Here's how the part is built. I have some questions about the finished solid (model axes, mm). A direction names the side the tool comes from. Give positions to 0.01 mm unless a question says otherwise; leave off trailing zeros. Write each loop counter-clockwise with the first axis right and the second up, starting at its lowest first coordinate (ties: lowest second). Pieces come first, ordered by that corner, then holes. Notation, with made-up numbers: M 24,-8 L 51,-8 A9 ccw 51,8 Z; hole C -21,-37.75 d9. An arc over 180 degrees is marked long. Answer as CSV lines item,"result". Start each with the question number.
Q1. Thinking about a two-plate mould opening in Y: for faces 3 (the cylindrical face through (124.178, 85.837, 6.788)), 4 (the flat face through (69, 0, 6)), 5 (the cylindrical face through (12.522, 85.837, 6.788)), 6 (the flat face through (69, 55, 12.7)), which applies, +Y half, -Y half, draft (parallel to the pull), parting line (faces both ways), or undercut?
Q2. On a 3-axis mill with a long thin cutter (end or side, diameter ignored), from which of +Z, -Z, +X, -X, +Y, -Y can I reach the whole of each face in a straight line? I mean faces 1 (the cylindrical face through (22.38, 12.88, 5.91)), 2 (the flat face through (0, 69, 6)). Say none if no direction works.
Q3. Suppose I cut it at D-D (x = 88). Write out the boundary of the cut face in (y, z).
Q4. For pin 1 (2 mm diameter, centred on x = 64, z = 2.5, fed in from +Y); pin 2 (2.5 mm diameter, centred on y = 83.866, z = 6.35, fed in from -X); pin 3 (3.5 mm diameter, centred on x = 24.35, z = 6.35, fed in from +Y), each with a flat end and sliding along its axis, tell me the tip position at first contact or that it passes through.
Q5. If I drill on line 1 along X through (y, z) = (8.5, 6.35); line 2 along Y through (x, z) = (115, 6); line 3 along Y through (x, z) = (121.75, 6.35), over which ranges is the centre line in solid material (lowest first)?
Q6. Suppose I cut it at A-A (y = 110.5). Write out the boundary of the cut face in (x, z).
Q7. Suppose I cut it at C-C (x = 127.5). Write out the boundary of the cut face in (y, z).
Q8. Suppose I cut it at B-B (z = 11). Write out the boundary of the cut face in (x, y).
```python
from build123d import *

# Parameters (mm, degrees)
BOSS_EXTRUDE1_DEPTH        = 12.7
F_10_32_TAPPED_HOLE2_D     = 4.0386
F_10_32_TAPPED_HOLE2_DEPTH = 25.4
F_10_32_TAPPED_HOLE2_TIP   = 1.213317848


with BuildPart() as part:
    # Sketch1 → Boss-Extrude1 (new body)
    with BuildSketch(Plane.XY):
        with BuildLine():
            Line((0, 0), (0, 140))
            Line((0, 140), (2.7, 140))
            ThreePointArc((2.7, 140), (68.35, 90.722783973), (134, 140))
            Line((134, 140), (136.7, 140))
            Line((136.7, 140), (136.7, 0))
            Line((136.7, 0), (0, 0))
        make_face()
    extrude(amount=BOSS_EXTRUDE1_DEPTH)

    # Sketch3 → #10-32 Tapped Hole1 (revolve, cut)
    with BuildSketch(Plane(origin=(136.7, 83.866, 6.35), x_dir=(0, 0, -1), z_dir=(0, 1, 0))):
        Polygon((0, 0), (0, 26.613317848), (2.0193, 25.4), (2.0193, 0), align=None)
    f_10_32_tapped_hole1 = revolve(axis=Axis((143.05, 83.866, 6.35), (-1, 0, 0)), mode=Mode.SUBTRACT)

    # Mirror3: #10-32 Tapped Hole1 across plane
    add(f_10_32_tapped_hole1.mirror(Plane(origin=(68.35, 0, 0), x_dir=(0, 0, 1), z_dir=(1, 0, 0))), mode=Mode.SUBTRACT)

    # #10-32 Tapped Hole2
    with Locations(Plane(origin=(112.35, 0, 6.35), x_dir=(0, 0, -1), z_dir=(0, -1, 0))):
        with Locations((0, 0), (0, -88)):
            Hole(F_10_32_TAPPED_HOLE2_D / 2, depth=F_10_32_TAPPED_HOLE2_DEPTH)
            with Locations((0, 0, -(F_10_32_TAPPED_HOLE2_DEPTH + F_10_32_TAPPED_HOLE2_TIP / 2))):  # 118° drill point
                Cone(0, F_10_32_TAPPED_HOLE2_D / 2, F_10_32_TAPPED_HOLE2_TIP, mode=Mode.SUBTRACT)


solid = part.part
```
Resolved:
1,face 3,"undercut"
1,face 4,"-Y half"
1,face 5,"undercut"
1,face 6,"draft"
2,face 1,"-Y"
2,face 2,"+Z, -Z, -X, +Y, -Y"
3,outline,"M 0,0 L 93.61,0 L 93.61,12.7 L 0,12.7 Z"
4,pin 1,"y = 90.93"
4,pin 2,"x = 25.86"
4,pin 3,"y = 108.29"
5,line 1,"0 to 22.33, 26.37 to 110.33, 114.37 to 136.7"
5,line 2,"0 to 81.88, 85.85 to 109.11"
5,line 3,"0 to 81.85, 85.89 to 116.4"
6,outline,"M 0,0 L 20.25,0 L 20.25,12.7 L 0,12.7 Z; M 116.45,0 L 136.7,0 L 136.7,12.7 L 116.45,12.7 Z"
7,outline,"M 0,0 L 124.8,0 L 124.8,12.7 L 0,12.7 Z; hole C 83.87,6.35 d4.04"
8,outline,"M 0,0 L 136.7,0 L 136.7,140 L 134,140 A68.37 cw 2.7,140 L 0,140 Z"
